Answer from the drawing. Dimensions are ordinates in mm from the lowest x, y and z of the part. A direction names the side the tool comes from. Give positions to 0.01 mm unless a question says otherwise; leave off trailing zeros. Loops run counter-clockwise (first coordinate to the right, second up) from the corner with the lowest first, then second, coordinate; pieces in that order, holes last.
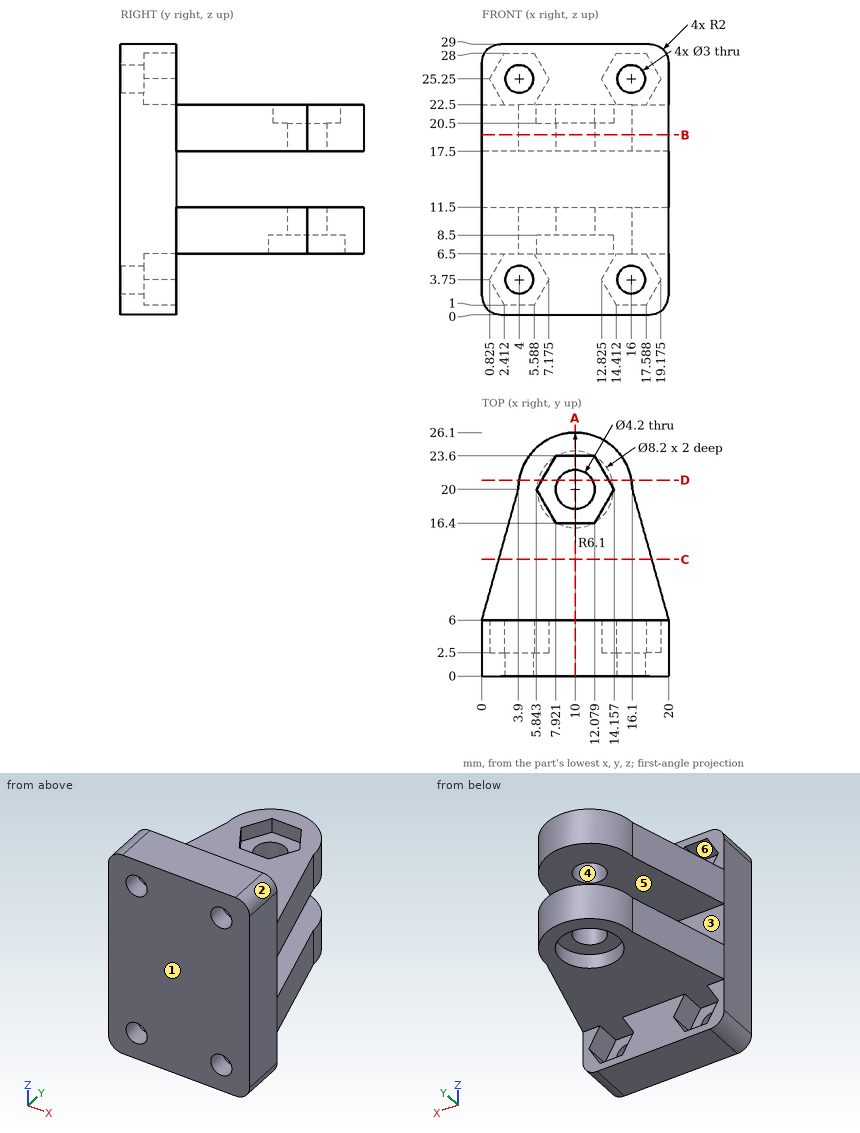
Item 1: Find section C-C, the plane y = 12.5. Write down the section's boundary in (x, z), plus the area to 3 significant figures.
Item 2: For the marked faces 4, 5 and 6, determine the directions among +Z, -Z, +X, -X, +Y, -Y from which every point of the face is accessible in a straight line to the end or side of a thin tool.
Item 3: Find section D-D, the plane y = 21. Write down the section's boundary in (x, z).
Item 4: Find section A-A, the plane x = 10. Write down the section's boundary in (y, z).
Item 5: Find section B-B, the plane z = 19.25. Write down the section's boundary in (x, y).
Item 6: Determine the mould class of the marked faces 1, 2 and 3 for opening direction Z: released by +Z, released by -Z, zero draft, split by the parting line, or undercut.
Item 7: Consider line 1 (X direction, y = 1.15, z = 3.75); line 2 (Z direction, x = 4, y = 1.95); line 3 (Z direction, x = 7, y = 18.5). Determine where each line is inside the solid, lowest interval first.
Item 8: Flat-ended cylindrical pins translate along their axes: pin 1 Ø6 at (x, y) = (10, 14.5) entering from -Z; pin 2 Ø4 at (x, z) = (4, 25.25) entering from +Y; pin 3 Ø6 at (x, y) = (6, 17.5) entering from +Z; pin 4 Ø1.8 at (x, z) = (16, 25.25) entering from -Y. Find the tip coordinate at first contact, or state that the pin passes through.
Ans:
1. outline: (1.81, 6.5) - (18.19, 6.5) - (18.19, 11.5) - (1.81, 11.5) - close; (1.81, 17.5) - (18.19, 17.5) - (18.19, 22.5) - (1.81, 22.5) - close
1. area: 164 mm2
2. face 4: +Z, -Z
2. face 5: +X, -X, +Y
2. face 6: +Y
3. outline: (3.98, 6.5) - (6.02, 6.5) - (6.02, 8.5) - (8.15, 8.5) - (8.15, 11.5) - (3.98, 11.5) - close; (3.98, 17.5) - (8.15, 17.5) - (8.15, 20.5) - (6.42, 20.5) - (6.42, 22.5) - (3.98, 22.5) - close; (11.85, 8.5) - (13.98, 8.5) - (13.98, 6.5) - (16.02, 6.5) - (16.02, 11.5) - (11.85, 11.5) - close; (11.85, 17.5) - (16.02, 17.5) - (16.02, 22.5) - (13.58, 22.5) - (13.58, 20.5) - (11.85, 20.5) - close
4. outline: (0, 0) - (6, 0) - (6, 6.5) - (15.9, 6.5) - (15.9, 8.5) - (17.9, 8.5) - (17.9, 11.5) - (6, 11.5) - (6, 17.5) - (17.9, 17.5) - (17.9, 20.5) - (16.4, 20.5) - (16.4, 22.5) - (6, 22.5) - (6, 29) - (0, 29) - close; (22.1, 8.5) - (24.1, 8.5) - (24.1, 6.5) - (26.1, 6.5) - (26.1, 11.5) - (22.1, 11.5) - close; (22.1, 17.5) - (26.1, 17.5) - (26.1, 22.5) - (23.6, 22.5) - (23.6, 20.5) - (22.1, 20.5) - close
5. outline: (0, 0) - (20, 0) - (20, 6) - (16.1, 20) arc R6.1 ccw to (3.9, 20) - (0, 6) - close; hole circle Ø4.2 at (10, 20)
6. face 1: zero draft
6. face 2: released by +Z
6. face 3: undercut
7. line 1: x = 0 to 2.5, 5.5 to 14.5, 17.5 to 20
7. line 2: z = 0 to 2.25, 5.25 to 23.75, 26.75 to 29
7. line 3: z = 8.5 to 11.5, 17.5 to 20.5
8. pin 1: stops at z = 6.5
8. pin 2: stops at y = 2.5
8. pin 3: stops at z = 22.5
8. pin 4: passes through
